Input: part model. Units: mm. Frame: model coordinates. A direction names the side the tool comes from. Round coordinates to 2 decimals unless told otherwise and drop trailing zeros. Loops run counter-clockwise (first coordinate to the right, second up) from the corner with the lowest first, then second, coordinate; pieces in that order, holes last. Notation, with made-up numbers: M -22,61 L 17,61 A23 cw 17,92 Z; hole C 42.5,-1.5 d4. An arc over 180 degrees is marked long. Use one line per item in the form item = value. Start each with the question number.
Q1. First-contact query: P1, Ø2.5, axis at y = 354, z = 461, coming from the +X side. Flat tip, straight axial feed; report the tip coordinate or a pass-through.
Q2. Access query for faces 1 (the flat face through (-8, 254, 464.499)), 2 (the flat face through (-8, 254, 455.499)). Directions: +Z, -Z, +X, -X, +Y, -Y. A direction counts if a zero-diameter tool reaches every point of the face in a straight line with its end or side. Return the directions, or none.
Q3. Ray query, line 1 along Y through (x, z) = (-7.5, 463.95); line 2 along Z through (x, y) = (-8.5, 180); line 3 along X through (y, z) = (113.5, 456.5). Return the intervals inside material, ascending.
Q4. Section query A-A, the plane y = 206.5. Output: boundary loops of the cut face in (x, z), and give its area (3 significant figures).
Q5. Mould query, pull axis Z, two halves, no side actions, for faces 3 (the flat face through (-8, 254, 454.499)), 4 (the flat face through (-14, 254, 460)), 5 (the flat face through (-15, 248, 460)). Classes: pulls with the +Z half, pulls with the -Z half, needs draft (parallel to the pull), parting line crosses it, or undercut.
```python
from build123d import *

# Parameters (mm, degrees)
SKETCH_1_W          = 15
SKETCH_1_H          = 475.958242536
SKETCH_1_R          = 1.6
EXTRUDE_1_DEPTH     = 10
SKETCH_2_W          = 15
SKETCH_2_H          = 25.958242536
CUT_EXTRUDE_1_DEPTH = 100
SKETCH_4_R          = 1.6
CUT_EXTRUDE_2_DEPTH = 15
SKETCH_5_W          = 13
SKETCH_5_H          = 8
CUT_EXTRUDE_3_DEPTH = 1000


with BuildPart() as part:
    # ｽｹｯﾁ1 → ﾎﾞｽ - 押し出し1 (new body)
    with BuildSketch(Plane.XY.offset(464.498723907)):
        with Locations((-7.5, 237.979121268)):
            Rectangle(SKETCH_1_W, SKETCH_1_H)
        with Locations((-7.5, 468.458242536)):
            Circle(SKETCH_1_R, mode=Mode.SUBTRACT)
        with Locations((-7.5, 149.274909628)):
            Circle(SKETCH_1_R, mode=Mode.SUBTRACT)
    extrude(amount=-EXTRUDE_1_DEPTH)

    # ｽｹｯﾁ2 → ｶｯﾄ - 押し出し1 (cut)
    with BuildSketch(Plane.XY.offset(464.498723907)):
        with Locations((-7.5, 12.979121268)):
            Rectangle(SKETCH_2_W, SKETCH_2_H)
    extrude(amount=-CUT_EXTRUDE_1_DEPTH, mode=Mode.SUBTRACT)

    # ｽｹｯﾁ4 → ｶｯﾄ - 押し出し2 (cut)
    with BuildSketch(Plane.ZY.offset(15)):
        with Locations(Location((459.498723907, 136.774909628, 0), (0, 0, 270))):
            Circle(SKETCH_4_R)
    extrude(amount=-CUT_EXTRUDE_2_DEPTH, mode=Mode.SUBTRACT)

    # ｽｹｯﾁ5 → ｶｯﾄ - 押し出し3 (cut)
    with BuildSketch(Plane(origin=(0, 475.958242536, 0), x_dir=(1, 0, 0), z_dir=(0, 1, 0))):
        with Locations((-7.5, -459.498723907)):
            Rectangle(SKETCH_5_W, SKETCH_5_H)
    extrude(amount=-CUT_EXTRUDE_3_DEPTH, mode=Mode.SUBTRACT)


solid = part.part
```
Results found:
q1.P1 = 0
q2.face_1 = +Z, +X, -X, +Y, -Y
q2.face_2 = +Y, -Y
q3.line_1 = 25.96 to 147.67, 150.87 to 466.86, 470.06 to 475.96
q3.line_2 = 454.5 to 455.5, 463.5 to 464.5
q3.line_3 = -15 to -14, -1 to 0
q4.outline = M -15,454.5 L 0,454.5 L 0,464.5 L -15,464.5 Z; hole M -14,455.5 L -1,455.5 L -1,463.5 L -14,463.5 Z
q4.area = 46.0 mm²
q5.face_3 = pulls with the -Z half
q5.face_4 = undercut
q5.face_5 = needs draft
